Build history of the part. All positions in model axes, mm. A direction names the side the tool comes from. Coordinates: 2 decimals unless noted, no trailing zeros. Order: outer loops, then holes, each group sorted by start corner. A loop starts at its lowest first (then second) coordinate and runs counter-clockwise, first axis right, second up. Notation, with made-up numbers: (15.25, -15.5) - (58.25, -15.5) arc R11 ccw to (58.25, -9.5) - close; hole circle Ø6 at (79, 85). An arc over 180 degrees is marked (long way). Answer as CSV lines item,"result". Start each with the question number.
from build123d import *

# Parameters (mm, degrees)
F0_W           = 6
F0_H           = 3.3
F1_DEPTH       = 42.5
F3_D           = 3.3
F3_CSINK_D     = 6.72
F3_CSINK_ANGLE = 90


with BuildPart() as f1:
    # F0 (on Front) → F1 (new body, symmetric)
    with BuildSketch(Plane.XZ):
        Rectangle(F0_W, F0_H)
        Polygon((4.7, -3.35), (3, -1.65), (-3, -1.65), (-4.7, -3.35), align=None)
    extrude(amount=F1_DEPTH, both=True)

    # F3 (through all)
    with Locations(Plane(origin=(0, 0, -3.35), x_dir=(1, 0, 0), z_dir=(0, 0, -1))):
        with Locations((0, 0), (0, 35), (0, -35)):
            CounterSinkHole(F3_D / 2, F3_CSINK_D / 2, counter_sink_angle=F3_CSINK_ANGLE)


solid = f1.part
(1) Pull direction Y, two halves, no side cores. Call faces 4 (the cylindrical face through (1.216, -1.115, 0.028)), 5 (the cylindrical face through (-0.89, 33.61, 0.03)), 6 (the flat face through (3.86, -0.59, -2.51)), 7 (the flat face through (0, -42.5, -1)): +Y half, -Y half, draft (parallel to the pull), parting line (faces both ways), or undercut.
(2) Drop flat-ended pins along their axis: pin 1 Ø5.5 at (x, y) = (0, -35) entering from -Z; pin 2 Ø2 at (y, z) = (-27, -1) entering from -X; pin 3 Ø1.5 at (y, z) = (6, -0.5) entering from -X. Give the stop position or say it passes through.
(3) Band-saw the part on A-A on z = -2.4. List the corners of the cut face in (x, y), plus the area to 3 significant figures.
(4) Band-saw the part on B-B on x = 0. List the corners of the cut face in (y, z).
(5) Band-saw the part on D-D on y = 15. List the corners of the cut face in (x, z), plus the area to 3 significant figures.
(6) Probe L1, parallel to Y at x = 0, z = 0.15; L2, parallel to Y at x = -1.5, z = -3.1; L3, parallel to X at y = 16.5, z = 0.7. List the from-to ranges inside material, lowest first. Write a range as [from, to].
(7) Band-saw the part on C-C on y = 35. List the corners of the cut face in (x, z), plus the area to 3 significant figures.
(8) Which spindle directions (+Z, -Z, +X, -X, +Y, -Y) get a long thin tool onto all of the face, cutting with end or side? Do faces 1 (the cylindrical face through (-0.89, -36.39, 0.03)), 2 (the flat face through (-3, -1, 0)), 3 (the flat face through (3, -1, 0)). Say none if no direction does.
Filled in:
1,face 4,"undercut"
1,face 5,"undercut"
1,face 6,"draft"
1,face 7,"-Y half"
2,pin 1,"stops at z = -2.74"
2,pin 2,"stops at x = -3.35"
2,pin 3,"stops at x = -3"
3,outline,"(-3.75, -42.5) - (3.75, -42.5) - (3.75, 42.5) - (-3.75, 42.5) - close; hole circle Ø4.82 at (0, -35); hole circle Ø4.82 at (0, 0); hole circle Ø4.82 at (0, 35)"
3,area,"583 mm^2"
4,outline,"(-42.5, -3.35) - (-38.36, -3.35) - (-36.65, -1.64) - (-36.65, 1.65) - (-42.5, 1.65) - close; (-33.35, -1.64) - (-31.64, -3.35) - (-3.36, -3.35) - (-1.65, -1.64) - (-1.65, 1.65) - (-33.35, 1.65) - close; (1.65, -1.64) - (3.36, -3.35) - (31.64, -3.35) - (33.35, -1.64) - (33.35, 1.65) - (1.65, 1.65) - close; (36.65, -1.64) - (38.36, -3.35) - (42.5, -3.35) - (42.5, 1.65) - (36.65, 1.65) - close"
5,outline,"(-4.7, -3.35) - (4.7, -3.35) - (3, -1.65) - (3, 1.65) - (-3, 1.65) - (-3, -1.65) - close"
5,area,"32.9 mm^2"
6,L1,"y = [-42.5, -36.65], [-33.35, -1.65], [1.65, 33.35], [36.65, 42.5]"
6,L2,"y = [-42.5, -37.72], [-32.28, -2.72], [2.72, 32.28], [37.72, 42.5]"
6,L3,"x = [-3, 3]"
7,outline,"(-4.7, -3.35) - (-3.36, -3.35) - (-1.65, -1.64) - (-1.65, 1.65) - (-3, 1.65) - (-3, -1.65) - close; (1.65, -1.64) - (3.36, -3.35) - (4.7, -3.35) - (3, -1.65) - (3, 1.65) - (1.65, 1.65) - close"
7,area,"13.5 mm^2"
8,face 1,"+Z, -Z"
8,face 2,"+Z, -X, +Y, -Y"
8,face 3,"+Z, +X, +Y, -Y"
